Check sheet for the modelled part. Datum: model origin and axes. Units: mm. A direction names the side the tool comes from. Round coordinates to 2 decimals unless told otherwise and drop trailing zeros. Loops run counter-clockwise (first coordinate to the right, second up) from the corner with the lowest first, then second, coordinate; pieces in that order, holes last. Notation, with made-up numbers: (-29.5, -13) - (27.5, -13) arc R15 cw to (27.5, -3) - close; hole circle Ø5 at (-36.5, 61.5). An arc over 180 degrees is marked (long way). Put each result on its own line as item: value.
```python
from build123d import *

# Parameters (mm, degrees)
CROQUIS1_R              = 15
SALIENTE_EXTRUIR1_DEPTH = 23
CROQUIS2_R              = 7.85
CORTAR_EXTRUIR1_DEPTH   = 16
CROQUIS3_R              = 1.5
CORTAR_EXTRUIR2_DEPTH   = 16


with BuildPart() as part:
    # Croquis1 → Saliente-Extruir1 (new body)
    with BuildSketch(Plane.XY):
        Circle(CROQUIS1_R)
    extrude(amount=-SALIENTE_EXTRUIR1_DEPTH)

    # Croquis2 → Cortar-Extruir1 (cut)
    with BuildSketch(Plane.XY):
        Circle(CROQUIS2_R)
    extrude(amount=-CORTAR_EXTRUIR1_DEPTH, mode=Mode.SUBTRACT)

    # Croquis3 → Cortar-Extruir2 (cut)
    with BuildSketch(Plane(origin=(0, 0, -23), x_dir=(-1, 0, 0), z_dir=(0, 0, -1))):
        Circle(CROQUIS3_R)
    extrude(amount=-CORTAR_EXTRUIR2_DEPTH, mode=Mode.SUBTRACT)


solid = part.part
```
Item 1: Section check A-A on x = 0. Enter the section's corners in (y, z), then the cut area to 3 significant figures.
Filled sheet:
outline: (-15, -23) - (-1.5, -23) - (-1.5, -16) - (-7.85, -16) - (-7.85, 0) - (-15, 0) - close; (1.5, -23) - (15, -23) - (15, 0) - (7.85, 0) - (7.85, -16) - (1.5, -16) - close
area: 418 mm²
Item 2: Section check C-C on z = -16.75. Enter the section's corners in (x, y), then the cut area to 3 significant figures.
Filled sheet:
outline: circle Ø30 at (0, 0); hole circle Ø3 at (0, 0)
area: 700 mm²
Item 3: Go/stop test with flat-tipped pins: pin 1 (8 mm diameter, centred on x = 4, y = 1.5, fed in from +Z); pin 2 (2.5 mm diameter, centred on x = 0, y = 0, fed in from +Z); pin 3 (1.5 mm diameter, centred on x = 9.5, z = -3.5, fed in from -Y); pin 4 (12 mm diameter, centred on y = -7.5, z = -8, fed in from +X). Record where each tip stops, or that it passes through.
Filled sheet:
pin 1: z = 0
pin 2: through
pin 3: y = -12.18
pin 4: x = 14.92
Item 4: Section check D-D on y = 2.5. Enter the section's corners in (x, z), then the cut area to 3 significant figures.
Filled sheet:
outline: (-14.79, -23) - (14.79, -23) - (14.79, 0) - (7.44, 0) - (7.44, -16) - (-7.44, -16) - (-7.44, 0) - (-14.79, 0) - close
area: 442 mm²
Item 5: Section check B-B on y = -0.75. Enter the section's corners in (x, z).
Filled sheet:
outline: (-14.98, -23) - (-1.3, -23) - (-1.3, -16) - (-7.81, -16) - (-7.81, 0) - (-14.98, 0) - close; (1.3, -23) - (14.98, -23) - (14.98, 0) - (7.81, 0) - (7.81, -16) - (1.3, -16) - close
Item 6: Release check for a two-part mould opening along Y. For faces 1 (the cylindrical face through (-5.786, 5.305, -7.888)), 2 (the cylindrical face through (-14.985, 0.66, -11.339)), 3 (the flat face through (3, 0, -23)) record: +Y half, -Y half, draft (parallel to the pull), parting line (faces both ways), or undercut.
Filled sheet:
face 1: undercut
face 2: parting line
face 3: draft
Item 7: Thickness scan on line 1 (Y direction, x = 0, z = -8); line 2 (Y direction, x = 0, z = -20.5); line 3 (Z direction, x = 0, y = 3). Record the ranges inside material, lowest first. Write a range as from..to.
Filled sheet:
line 1: -15..-7.85, 7.85..15
line 2: -15..-1.5, 1.5..15
line 3: -23..-16
Item 8: Tool access check on faces 4 (the cylindrical face through (1.5, 0.07, -19.55)), 5 (the flat face through (0, -2, -16)). Record the directions out of +Z, -Z, +X, -X, +Y, -Y that give a thin tool (end or side, any length) a straight path to the whole face; none if there is none.
Filled sheet:
face 4: +Z, -Z
face 5: +Z
